Could you check a few things on this drawing? It's one solid part, dimensions in mm from its lowest x, y, z. A direction names the side the tool comes from. Coordinates: 2 decimals unless noted, no trailing zeros. Order: outer loops, then holes, each group sorted by start corner. A loop starts at its lowest first (then second) coordinate and runs counter-clockwise, first axis right, second up.
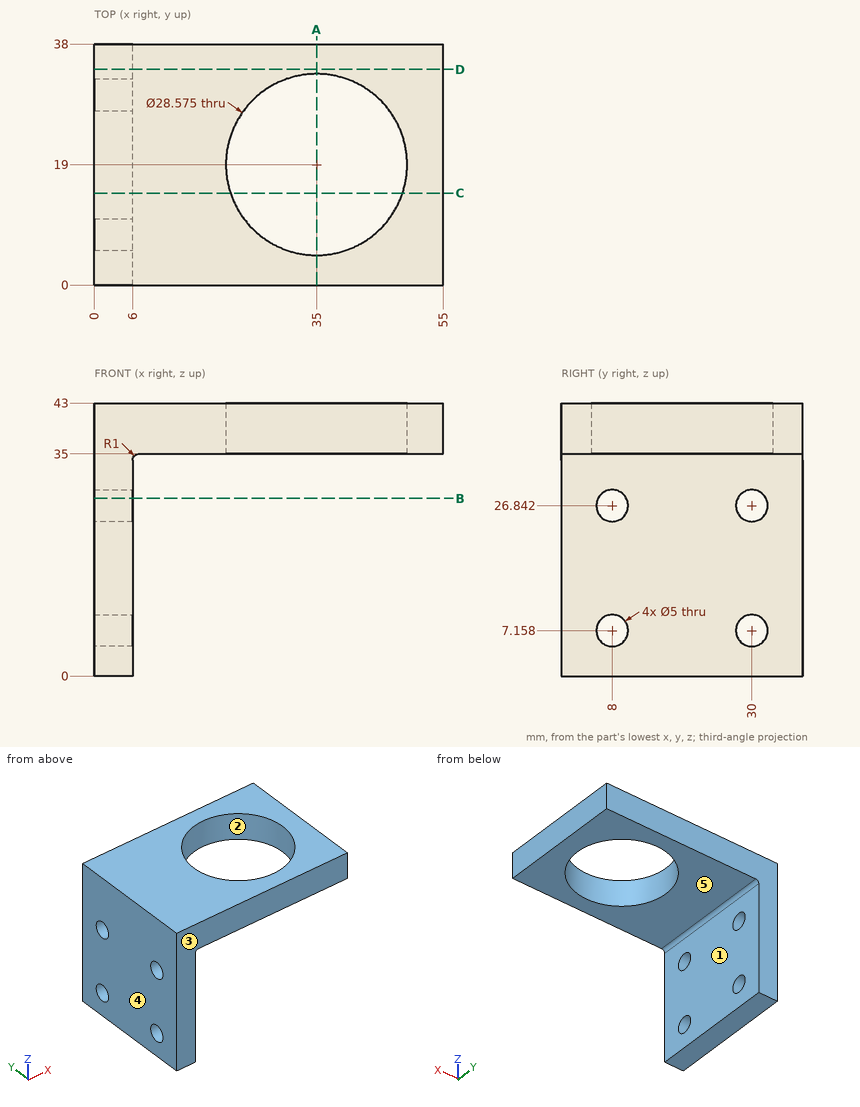
1. Imagine slicing it at D-D on y = 34. Please give me the cut outline in (x, z).
Completed:
outline: (0, 0) - (6, 0) - (6, 34) arc R1 cw to (7, 35) - (55, 35) - (55, 43) - (0, 43) - close
2. Thinking about a two-plate mould opening in Y: for the marked faces 1, 2 and 3, which applies, pulls with the +Y half, pulls with the -Y half, needs draft (parallel to the pull), parting line crosses it, or undercut?
Completed:
face 1: needs draft
face 2: undercut
face 3: pulls with the -Y half
3. I'm going to push flat-ended pins straight in: pin 1 (17 mm diameter, centred on y = 13, z = 19, fed in from +X); pin 2 (1 mm diameter, centred on x = 18, y = 30, fed in from -Z); pin 3 (17 mm diameter, centred on x = 35, y = 19, fed in from +Z). Where does each tip first touch, or does it pass through?
Completed:
pin 1: stops at x = 6
pin 2: stops at z = 35
pin 3: passes through
4. Imagine slicing it at C-C on y = 14.5. Please give me the cut outline in (x, z), then the cut area to 3 significant figures.
Completed:
outline: (0, 0) - (6, 0) - (6, 34) arc R1 cw to (7, 35) - (21.44, 35) - (21.44, 43) - (0, 43) - close; (48.56, 35) - (55, 35) - (55, 43) - (48.56, 43) - close
area: 433 mm2
5. Imagine slicing it at A-A on x = 35. Please give me the cut outline in (y, z), then the cut area to 3 significant figures.
Completed:
outline: (0, 35) - (4.71, 35) - (4.71, 43) - (0, 43) - close; (33.29, 35) - (38, 35) - (38, 43) - (33.29, 43) - close
area: 75.4 mm2
6. Imagine slicing it at B-B on z = 28. Please give me the cut outline in (x, y), then the cut area to 3 significant figures.
Completed:
outline: (0, 0) - (6, 0) - (6, 5.78) - (0, 5.78) - close; (0, 10.22) - (6, 10.22) - (6, 27.78) - (0, 27.78) - close; (0, 32.22) - (6, 32.22) - (6, 38) - (0, 38) - close
area: 175 mm2
7. On a 3-axis mill with a long thin cutter (end or side, diameter ignored), from which of +Z, -Z, +X, -X, +Y, -Y can I reach the whole of each face in a straight line? I mean the marked faces 4 and 5. Say none if no direction works.
Completed:
face 4: +Z, -Z, -X, +Y, -Y
face 5: -Z, +X, +Y, -Y
8. Please list where these lines run through material, in increasing order: probe 1 along Y at (x, z) = (35, 41); probe 2 along Z at (x, y) = (30.5, 33.5); probe 3 along X at (y, z) = (32, 17.5).
Completed:
probe 1: y = 0 to 4.71, 33.29 to 38
probe 2: z = 35 to 43
probe 3: x = 0 to 6
